Check sheet for the modelled part. Datum: model origin and axes. Units: mm. A direction names the side the tool comes from. Give positions to 0.01 mm unless a question says otherwise; leave off trailing zeros. Write each loop counter-clockwise with the first axis right and the second up, starting at its lowest first coordinate (ties: lowest second). Pieces come first, ordered by that corner, then holes. Notation, with made-up numbers: M 19.25,33.5 L 62.25,33.5 A26 ccw 62.25,47.5 Z; hole C 39.25,15.5 d10. An arc over 180 degrees is marked long. Use CSV: the item, a comma, the result in double quotes. Start each with the question number.
1. Cross-section at A-A, the plane x = 0. Enter the section's corners in (y, z).
2. Cross-section at B-B, the plane z = 2. Enter the section's corners in (x, y).
3. Cross-section at C-C, the plane x = 16.5. Enter the section's corners in (y, z), and give its area (3 significant figures).
4. Depth check by flat-ended pin: P1, Ø8, axis at x = -10, y = -2, coming from the -Z side; P2, Ø2.5, axis at y = 0, z = -7, coming from the +X side; P3, Ø1, axis at x = 16.5, y = 2.5, coming from the -Z side. Enter the tip coordinate at first touch or a pass-through.
5. Cross-section at D-D, the plane z = -7. Enter the section's corners in (x, y).
6. Access from +Z, -Z, +X, -X, +Y, -Y to the whole of each face (thin tool, end or side, straight path). Record for faces 5 (the face through (10.316, -7.91, -1.972)), 6 (the face through (-20.748, 0.11, 1.972)).
7. Scan lines: line 1 (Z direction, x = -5, y = 0); line 2 (Y direction, x = 0, z = -5.75); line 3 (X direction, y = 2, z = 1.5). Record each from-to range of solid material in increasing order.
8. Mould release check, pull along X, two halves, no side actions. Record for faces 1 (the face through (13.39, -8.49, 1.97)), 2 (the face through (1.42, -3.92, -9)), 3 (the face through (0.03, -4.98, -7.75)), 4 (the face through (0, 0, 0)): +X half, -X half, draft (parallel to the pull), parting line (faces both ways), or undercut.
from build123d import *

# Parameters (mm, degrees)
SKETCH1_R               = 2.5
BOSS_EXTRUDE1_DEPTH     = 4
SKETCH2_R               = 13
SKETCH2_R_2             = 11
EXTRUDE_THIN1_DEPTH     = 4
SKETCH3_R               = 6
SKETCH3_R_2             = 4
EXTRUDE_THIN2_DEPTH     = 9
CUT_EXTRUDE1_DEPTH      = 29.763040521
CUT_EXTRUDE1_DEPTH_BACK = 29.763040521
SKETCH4_R               = 0.75
CUT_EXTRUDE2_DEPTH      = 29.763040552
CUT_EXTRUDE2_DEPTH_BACK = 29.763040552
SKETCH5_R               = 0.75


with BuildPart() as part:
    # Sketch1 → Boss-Extrude1 (new body)
    with BuildSketch(Plane.XY):
        with BuildLine():
            Line((-20.660958904, 4.943407445), (-5.917808219, 12.133818273))
            ThreePointArc((-5.917808219, 12.133818273), (0, 13.5), (5.917808219, 12.133818273))
            Line((5.917808219, 12.133818273), (20.660958904, 4.943407445))
            ThreePointArc((20.660958904, 4.943407445), (23.75, 0), (20.660958904, -4.943407445))
            Line((20.660958904, -4.943407445), (5.917808219, -12.133818273))
            ThreePointArc((5.917808219, -12.133818273), (0, -13.5), (-5.917808219, -12.133818273))
            Line((-5.917808219, -12.133818273), (-20.660958904, -4.943407445))
            ThreePointArc((-20.660958904, -4.943407445), (-23.75, 0), (-20.660958904, 4.943407445))
        make_face()
        with Locations((-18.25, 0)):
            Circle(SKETCH1_R, mode=Mode.SUBTRACT)
        with Locations((18.25, 0)):
            Circle(SKETCH1_R, mode=Mode.SUBTRACT)
    extrude(amount=BOSS_EXTRUDE1_DEPTH)

    # Sketch2 → Extrude-Thin1 (add)
    with BuildSketch(Plane(origin=(0, 0, 0), x_dir=(-1, 0, 0), z_dir=(0, 0, -1))):
        Circle(SKETCH2_R)
        Circle(SKETCH2_R_2, mode=Mode.SUBTRACT)
    extrude(amount=EXTRUDE_THIN1_DEPTH)

    # Sketch3 → Extrude-Thin2 (add)
    with BuildSketch(Plane(origin=(0, 0, 0), x_dir=(-1, 0, 0), z_dir=(0, 0, -1))):
        Circle(SKETCH3_R)
        Circle(SKETCH3_R_2, mode=Mode.SUBTRACT)
    extrude(amount=EXTRUDE_THIN2_DEPTH)

    # Sketch4 → Cut-Extrude1 (cut, two sides: drawn at the far end of the back side and taken through both)
    with BuildSketch(Plane(origin=(0, 0, 0), x_dir=(0, 0, -1), z_dir=(1, 0, 0)).offset(-CUT_EXTRUDE1_DEPTH_BACK)):
        with Locations((7, 0)):
            Circle(SKETCH4_R)
    extrude(amount=CUT_EXTRUDE1_DEPTH + CUT_EXTRUDE1_DEPTH_BACK, mode=Mode.SUBTRACT)

    # Sketch5 → Cut-Extrude2 (cut, two sides: drawn at the far end of the back side and taken through both)
    with BuildSketch(Plane(origin=(0, 0, 0), x_dir=(1, 0, 0), z_dir=(0, 1, 0)).offset(-CUT_EXTRUDE2_DEPTH_BACK)):
        with Locations(Location((0, 7, 0), (0, 0, 270))):
            Circle(SKETCH5_R)
    extrude(amount=CUT_EXTRUDE2_DEPTH + CUT_EXTRUDE2_DEPTH_BACK, mode=Mode.SUBTRACT)


solid = part.part
Worked answers:
1,outline,"M -13.5,0 L -13,0 L -13,-4 L -11,-4 L -11,0 L -6,0 L -6,-6.25 L -4,-6.25 L -4,0 L 4,0 L 4,-6.25 L 6,-6.25 L 6,0 L 11,0 L 11,-4 L 13,-4 L 13,0 L 13.5,0 L 13.5,4 L -13.5,4 Z; M -6,-9 L -4,-9 L -4,-7.75 L -6,-7.75 Z; M 4,-9 L 6,-9 L 6,-7.75 L 4,-7.75 Z"
2,outline,"M -20.66,-4.94 L -5.92,-12.13 A13.5 ccw 5.92,-12.13 L 20.66,-4.94 A5.5 ccw 20.66,4.94 L 5.92,12.13 A13.5 ccw -5.92,12.13 L -20.66,4.94 A5.5 ccw Z; hole C -18.25,0 d5; hole C 18.25,0 d5"
3,outline,"M -6.97,0 L -1.79,0 L -1.79,4 L -6.97,4 Z; M 1.79,0 L 6.97,0 L 6.97,4 L 1.79,4 Z"
3,area,"41.5 mm^2"
4,P1,"stops at z = -4"
4,P2,"stops at x = 6"
4,P3,"stops at z = 0"
5,outline,"M -5.95,-0.75 A6 ccw -0.75,-5.95 L -0.75,-3.93 A4 cw -3.93,-0.75 Z; M -5.95,0.75 L -3.93,0.75 A4 cw -0.75,3.93 L -0.75,5.95 A6 ccw Z; M 0.75,-5.95 A6 ccw 5.95,-0.75 L 3.93,-0.75 A4 cw 0.75,-3.93 Z; M 0.75,3.93 A4 cw 3.93,0.75 L 5.95,0.75 A6 ccw 0.75,5.95 Z"
6,face 5,"-Z"
6,face 6,"+Z, -Z"
7,line 1,"z = -9 to -7.75, -6.25 to 4"
7,line 2,"y = -6 to -4, 4 to 6"
7,line 3,"x = -23.37 to -19.75, -16.75 to 16.75, 19.75 to 23.37"
8,face 1,"+X half"
8,face 2,"draft"
8,face 3,"undercut"
8,face 4,"undercut"
